Here's how the part is built. I have some questions about the finished solid (model axes, mm). Face numbers are marked on the shaded views. A direction names the side the tool comes from. Round coordinates to 2 decimals unless told otherwise and drop trailing zeros. Order: outer loops, then holes, each group sorted by start corner. A loop starts at its lowest first (then second) coordinate and runs counter-clockwise, first axis right, second up. Notation, with made-up numbers: (1, -7) -> (20, -7) arc R10 cw to (20, 9) -> close; hole circle Ø10 at (60, 67.5). An arc over 180 degrees is marked (long way). One line per item, written item: value.
```python
from build123d import *

# Parameters (mm, degrees)
SKETCH2_R          = 5
CUT_EXTRUDE1_DEPTH = 56
CIRPATTERN1_COUNT  = 4


with BuildPart() as part:
    # Sketch1 → Revolve1 (revolve)
    with BuildSketch(Plane.XY):
        Polygon((11.25, -75.117525247), (22.5, -75.117525247), (32.5, -33.117525247), (26.5, -33.117525247), (19, -63.117525247), (11, -63.117525247), align=None)
    revolve(axis=Axis((0, 54.787552818, 0), (0, -1, 0)))

    # Sketch2 → Cut-Extrude1 (cut)
    with BuildSketch(Plane.XY):
        with Locations((0, -33.117525247)):
            Circle(SKETCH2_R)
    cut_extrude1 = extrude(amount=-CUT_EXTRUDE1_DEPTH, mode=Mode.SUBTRACT)

    # CirPattern1: Cut-Extrude1 ×4 about axis
    cirpattern1_axis = Axis((0, -63.117525247, 0), (0, -1, 0))
    for i in range(1, CIRPATTERN1_COUNT):
        add(cut_extrude1.rotate(cirpattern1_axis, i * 360 / CIRPATTERN1_COUNT), mode=Mode.SUBTRACT)


solid = part.part
```
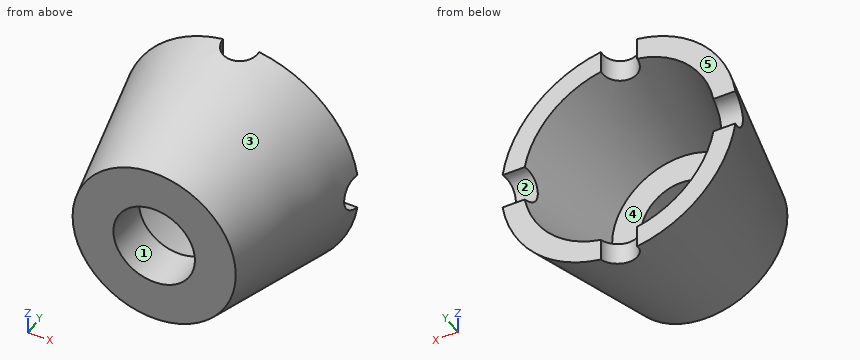
Q1. If we mould it in two halves opening along X, with no side actions, what happens to the marked faces 1, 2 and 3? For each: pulls with the +X half, pulls with the -X half, needs draft (parallel to the pull), parting line crosses it, or undercut.
Answers:
face 1: undercut
face 2: needs draft
face 3: parting line crosses it
Q2. For P1, Ø10, axis at x = -19, y = -56.5, coming from the +Z side; P2, Ø1.5, axis at y = -69.5, z = -12.5, coming from the +X side; P3, Ø2, axis at y = -48.5, z = 3, coming from the +X side, each with a flat end and sliding along its axis, tell me the tip position at first contact or that it passes through.
Answers:
P1: z = 23.31
P2: x = 20.79
P3: x = 28.94
Q3. I want a section at D-D on y = -68.5. Write out the boundary of the cut face in (x, z).
Answers:
outline: circle Ø48.15 at (0, 0); hole circle Ø22.22 at (0, 0)
Q4. I want a section at A-A on y = -35.5. Write out the boundary of the cut face in (x, z), then the cut area to 3 significant figures.
Answers:
outline: (-31.63, -4.4) arc R31.93 ccw to (-4.4, -31.63) -> (-4.4, -25.53) arc R25.9 cw to (-25.53, -4.4) -> close; (-31.63, 4.4) -> (-25.53, 4.4) arc R25.9 cw to (-4.4, 25.53) -> (-4.4, 31.63) arc R31.93 ccw to start; (4.4, -31.63) arc R31.93 ccw to (31.63, -4.4) -> (25.53, -4.4) arc R25.9 cw to (4.4, -25.53) -> close; (4.4, 25.53) arc R25.9 cw to (25.53, 4.4) -> (31.63, 4.4) arc R31.93 ccw to (4.4, 31.63) -> close
area: 883 mm2
Q5. I want a section at B-B on x = 0. Write out the boundary of the cut face in (y, z), then the cut area to 3 significant figures.
Answers:
outline: (-75.12, -22.5) -> (-38.12, -31.31) -> (-38.12, -25.25) -> (-63.12, -19) -> (-63.12, -11) -> (-75.12, -11.25) -> close; (-75.12, 11.25) -> (-63.12, 11) -> (-63.12, 19) -> (-38.12, 25.25) -> (-38.12, 31.31) -> (-75.12, 22.5) -> close
area: 618 mm2
Q6. Which directions (+Z, -Z, +X, -X, +Y, -Y) give clear straight access to the entire face, cutting with the end or side of a thin tool? Please do the marked faces 4 and 5.
Answers:
face 4: +Y
face 5: +Z, -Z, +X, -X, +Y
Q7. I want a section at C-C on z = 0. Write out the boundary of the cut face in (x, y).
Answers:
outline: (-31.31, -38.12) -> (-22.5, -75.12) -> (-11.25, -75.12) -> (-11, -63.12) -> (-19, -63.12) -> (-25.25, -38.12) -> close; (11, -63.12) -> (11.25, -75.12) -> (22.5, -75.12) -> (31.31, -38.12) -> (25.25, -38.12) -> (19, -63.12) -> close
Q8. I need wall thicknesses on line 1 along X through (y, z) = (-42.5, -2); line 2 along Y through (x, z) = (10.5, -8); line 3 along X through (y, z) = (-70.5, -3.5). Which ranges of each line are inside material? Lowest first, please.
Answers:
line 1: -30.2 to -24.07, 24.07 to 30.2
line 2: -75.12 to -63.12
line 3: -23.34 to -10.59, 10.59 to 23.34
